Input: part model. Units: mm. Frame: model coordinates. A direction names the side the tool comes from. Give positions to 0.01 mm unless a question says otherwise; leave off trailing zeros. Loops run counter-clockwise (first coordinate to the right, second up) from the corner with the lowest first, then second, coordinate; pieces in that order, holes last. Notation, with made-up numbers: (46.5, 41.25) -> (93.5, 41.25) arc R19 ccw to (93.5, 58.25) -> close; hole circle Ø10 at (79, -27). An arc over 180 degrees is marked (long way). Answer as a JSON object with one key per item and string values.
```python
from build123d import *

# Parameters (mm, degrees)
F1_DEPTH = 40
F2_DEPTH = 55
F3_DEPTH = 80
F4_DEPTH = 20
F5_W     = 25
F5_H     = 15
F6_DEPTH = 75
F8_DEPTH = 35


with BuildPart() as f1:
    # F0 (on Top) → F1 (new body)
    with BuildSketch(Plane.XY):
        Polygon((0, 50), (0, 0), (9, 15), (30, 50), (30, 87.5), align=None)
    extrude(amount=F1_DEPTH)

    # F0 (on Top) → F2 (join)
    with BuildSketch(Plane.XY):
        Polygon((0, 100), (0, 50), (30, 87.5), (40, 100), align=None)
    extrude(amount=F2_DEPTH)

    # F0 (on Top) → F3 (join)
    with BuildSketch(Plane.XY):
        Polygon((0, 135), (0, 100), (40, 100), (70, 100), (70, 135), align=None)
    extrude(amount=F3_DEPTH)

    # F0 (on Top) → F4 (join)
    with BuildSketch(Plane.XY):
        Polygon((30, 50), (9, 15), (70, 15), (70, 100), (40, 100), (30, 87.5), align=None)
    extrude(amount=F4_DEPTH)

    # F5 (on face) → F6 (cut)
    with BuildSketch(Plane.XY.offset(80)):
        with Locations((57.5, 117.5)):
            Rectangle(F5_W, F5_H)
    extrude(amount=-F6_DEPTH, mode=Mode.SUBTRACT)

    # F7 (on face) → F8 (cut, through all)
    with BuildSketch(Plane(origin=(0, 135, 0), x_dir=(-1, 0, 0), z_dir=(0, 1, 0))):
        Polygon((-70, 80), (-70, 35), (-40, 80), align=None)
    extrude(amount=-F8_DEPTH, mode=Mode.SUBTRACT)


solid = f1.part
```
Q1. Section D-D, the plane x = 53. Return the cut outline in (y, z).
Evaluation:
{"outline": "(15, 0) -> (135, 0) -> (135, 60.5) -> (125, 60.5) -> (125, 5) -> (110, 5) -> (110, 60.5) -> (100, 60.5) -> (100, 20) -> (15, 20) -> close"}
Q2. Pin query (flat end, axial travel): pin 1 (5 mm diameter, centred on x = 30, z = 70, fed in from -Y); pin 2 (4.5 mm diameter, centred on y = 120.5, z = 34, fed in from +X); pin 3 (7.5 mm diameter, centred on x = 53.5, y = 114.5, fed in from +Z). Return the tip coordinate at first contact, or that it passes through.
Evaluation:
{"pin 1": "stops at y = 100", "pin 2": "stops at x = 45", "pin 3": "stops at z = 5"}
Q3. Ray query, line 1 along Y through (x, z) = (53, 56); line 2 along Z through (x, y) = (23.5, 30); line 3 along Y through (x, z) = (15.5, 7). Return the intervals inside material, ascending.
Evaluation:
{"line 1": "y = 100 to 110, 125 to 135", "line 2": "z = 0 to 20", "line 3": "y = 15 to 135"}
Q4. Section A-A, the plane z = 25.5. Return the cut outline in (x, y).
Evaluation:
{"outline": "(0, 0) -> (30, 50) -> (30, 87.5) -> (40, 100) -> (70, 100) -> (70, 110) -> (45, 110) -> (45, 125) -> (70, 125) -> (70, 135) -> (0, 135) -> close"}
Q5. Draft query along Y for faces 1 (the flat face through (45, 117, 39)), 2 (the flat face through (39, 15, 10)), 3 (the flat face through (35, 68, 0)). Return one class per face: +Y half, -Y half, draft (parallel to the pull), parting line (faces both ways), or undercut.
Evaluation:
{"face 1": "undercut", "face 2": "-Y half", "face 3": "draft"}
Q6. Section C-C, the plane y = 76.5. Return the cut outline in (x, z), then the cut area to 3 significant figures.
Evaluation:
{"outline": "(0, 0) -> (70, 0) -> (70, 20) -> (30, 20) -> (30, 40) -> (21.2, 40) -> (21.2, 55) -> (0, 55) -> close", "area": "2,320 mm2"}
Q7. Section B-B, the plane x = 63. Return the cut outline in (y, z).
Evaluation:
{"outline": "(15, 0) -> (135, 0) -> (135, 45.5) -> (125, 45.5) -> (125, 5) -> (110, 5) -> (110, 45.5) -> (100, 45.5) -> (100, 20) -> (15, 20) -> close"}
Q8. Access query for faces 4 (the flat face through (46, 58, 20)), 5 (the flat face through (15, 81, 55)), 6 (the flat face through (57, 118, 5)), 7 (the flat face through (20, 118, 80)). Directions: +Z, -Z, +X, -X, +Y, -Y. A direction counts if a zero-diameter tool reaches every point of the face in a straight line with its end or side. Return the directions, or none.
Evaluation:
{"face 4": "+Z, +X, -Y", "face 5": "+Z, +X, -X, -Y", "face 6": "+Z, +X", "face 7": "+Z, +X, -X, +Y, -Y"}
